Verification items for the finished model (mm, model axes). A direction names the side the tool comes from. Coordinates: 2 decimals unless noted, no trailing zeros. Write each loop counter-clockwise with the first axis right and the second up, starting at its lowest first coordinate (ties: lowest second). Pieces come first, ordered by that corner, then holes. Notation, with made-up numbers: (-20.5, 20.5) -> (27.5, 20.5) arc R18 ccw to (27.5, 37.5) -> close; hole circle Ø7 at (32.5, 45.25). An arc over 180 degrees is marked (long way). Use CSV: the item, a comma, the result in double quotes.
```python
from build123d import *

# Parameters (mm, degrees)
BOSS_EXTRUDE1_DEPTH = 609.6
SHELL1_T            = -7.62


with BuildPart() as part:
    # Sketch1 → Boss-Extrude1 (new body)
    with BuildSketch(Plane(origin=(0, 0, 0), x_dir=(1, 0, 0), z_dir=(0, 1, 0))):
        with BuildLine():
            Line((0, 0), (381, 0))
            ThreePointArc((381, 0), (392.440846298, 4.738953702), (397.1798, 16.1798))
            Line((397.1798, 16.1798), (397.1798, 244.7798))
            ThreePointArc((397.1798, 244.7798), (392.440846298, 256.220646298), (381, 260.9596))
            Line((381, 260.9596), (0, 260.9596))
            ThreePointArc((0, 260.9596), (-11.440846298, 256.220646298), (-16.1798, 244.7798))
            Line((-16.1798, 244.7798), (-16.1798, 16.1798))
            ThreePointArc((-16.1798, 16.1798), (-11.440846298, 4.738953702), (0, 0))
        make_face()
    extrude(amount=-BOSS_EXTRUDE1_DEPTH)

    # Shell1
    shell1_openings = [part.faces().sort_by_distance(p)[0] for p in [
        (190.5, 0, -130.4798),
    ]]
    offset(amount=SHELL1_T, openings=shell1_openings, kind=Kind.INTERSECTION)


solid = part.part
```
1) Mould release check, pull along Z, two halves, no side actions. Record for faces 3 (the flat face through (193, -301, -260.96)), 4 (the flat face through (397.18, -301, -129)), 5 (the flat face through (188, -601.98, -132)): released by +Z, released by -Z, zero draft, split by the parting line, or undercut.
Return value:
face 3,"released by -Z"
face 4,"zero draft"
face 5,"undercut"
2) Cross-section at A-A (y = -82). Record the boundary of the cut face in (x, z), plus the area to 3 significant figures.
Return value:
outline,"(-16.18, -244.78) arc R16.18 ccw to (0, -260.96) -> (381, -260.96) arc R16.18 ccw to (397.18, -244.78) -> (397.18, -16.18) arc R16.18 ccw to (381, 0) -> (0, 0) arc R16.18 ccw to (-16.18, -16.18) -> close; hole (-8.56, -244.78) arc R8.56 ccw to (0, -253.34) -> (381, -253.34) arc R8.56 ccw to (389.56, -244.78) -> (389.56, -16.18) arc R8.56 ccw to (381, -7.62) -> (0, -7.62) arc R8.56 ccw to (-8.56, -16.18) -> close"
area,"9,880 mm2"
3) Scan lines: L1, parallel to Z at x = 289.5, y = -357.5; L2, parallel to X at y = -221, z = -105; L3, parallel to Y at x = 370, z = -20. Record each from-to range of solid material in increasing order.
Return value:
L1,"-260.96 to -253.34, -7.62 to 0"
L2,"-16.18 to -8.56, 389.56 to 397.18"
L3,"-609.6 to -601.98"
4) Cross-section at C-C (z = -75.5). Record the boundary of the cut face in (x, y).
Return value:
outline,"(-16.18, -609.6) -> (397.18, -609.6) -> (397.18, 0) -> (389.56, 0) -> (389.56, -601.98) -> (-8.56, -601.98) -> (-8.56, 0) -> (-16.18, 0) -> close"
5) Cross-section at B-B (x = 357.5). Record the boundary of the cut face in (y, z), plus the area to 3 significant figures.
Return value:
outline,"(-609.6, -260.96) -> (0, -260.96) -> (0, -253.34) -> (-601.98, -253.34) -> (-601.98, -7.62) -> (0, -7.62) -> (0, 0) -> (-609.6, 0) -> close"
area,"11,200 mm2"
6) Set-up check for faces 1 (the cylindrical face through (392.57, -300.53, -256.09)), 2 (the flat face through (193, -297, -253.34)): record each of +Z, -Z, +X, -X, +Y, -Y from which the full face is reachable in a straight line by a thin tool's end or side.
Return value:
face 1,"-Z, +X, +Y, -Y"
face 2,"+Y"
